from build123d import *

# Parameters (mm, degrees)
F0_W        = 88.9
F0_H        = 165.1
F1_DEPTH    = 6.35
F2_DEPTH    = 25.4
F3_DEPTH    = 50.8
F4_R        = 6.34999
F5_SIZE2    = 12.7
F5_SIZE     = 12.7
F6_C1_SIZE2 = 12.7
F6_C1_SIZE  = 7.3323484187
F6_C2_SIZE2 = 7.3323484187
F6_C2_SIZE  = 12.7
F6_C3_SIZE2 = 7.3323484187
F6_C3_SIZE  = 12.7
F6_C4_SIZE2 = 7.3323484187
F6_C4_SIZE  = 12.7


# Not quite as in the source:
# - a fillet or chamfer is up to 0.001 mm smaller than in the source, because OpenCascade refuses the exact size


with BuildPart() as f1:
    # F0 (on Top) → F1 (new body)
    with BuildSketch(Plane.XY):
        with Locations((59.7539862376, 23.8323401288)):
            Rectangle(F0_W, F0_H)
        Polygon((21.6539862376, 61.9323401288), (21.6539862376, 100.0323401288), (59.7539862376, 100.0323401288), (97.8539862376, 100.0323401288), (97.8539862376, -14.2676598712), (97.8539862376, -52.3676598712), (59.7539862376, -52.3676598712), (21.6539862376, -52.3676598712), align=None, mode=Mode.SUBTRACT)
    extrude(amount=F1_DEPTH)

    # F0 (on Top) → F2 (join)
    with BuildSketch(Plane.XY):
        with BuildLine():
            Line((97.8539862376, 100.0323401288), (59.7539862376, 100.0323401288))
            Line((59.7539862376, 100.0323401288), (59.7539862376, 74.6323401288))
            ThreePointArc((59.7539862376, 74.6323401288), (56.0342423587, 65.6520840077), (47.0539862376, 61.9323401288))
            Line((47.0539862376, 61.9323401288), (21.6539862376, 61.9323401288))
            Line((21.6539862376, 61.9323401288), (21.6539862376, -52.3676598712))
            Line((21.6539862376, -52.3676598712), (59.7539862376, -52.3676598712))
            Line((59.7539862376, -52.3676598712), (59.7539862376, -26.9676598712))
            ThreePointArc((59.7539862376, -26.9676598712), (63.4737301166, -17.9874037501), (72.4539862376, -14.2676598712))
            Line((72.4539862376, -14.2676598712), (97.8539862376, -14.2676598712))
            Line((97.8539862376, -14.2676598712), (97.8539862376, 100.0323401288))
        make_face()
    extrude(amount=F2_DEPTH)

    # F0 (on Top) → F3 (join)
    with BuildSketch(Plane.XY):
        with BuildLine():
            Line((59.7539862376, 100.0323401288), (21.6539862376, 100.0323401288))
            Line((21.6539862376, 100.0323401288), (21.6539862376, 61.9323401288))
            Line((21.6539862376, 61.9323401288), (47.0539862376, 61.9323401288))
            ThreePointArc((47.0539862376, 61.9323401288), (56.0342423587, 65.6520840077), (59.7539862376, 74.6323401288))
            Line((59.7539862376, 74.6323401288), (59.7539862376, 100.0323401288))
        make_face()
        with BuildLine():
            Line((97.8539862376, -52.3676598712), (97.8539862376, -14.2676598712))
            Line((97.8539862376, -14.2676598712), (72.4539862376, -14.2676598712))
            ThreePointArc((72.4539862376, -14.2676598712), (63.4737301166, -17.9874037501), (59.7539862376, -26.9676598712))
            Line((59.7539862376, -26.9676598712), (59.7539862376, -52.3676598712))
            Line((59.7539862376, -52.3676598712), (97.8539862376, -52.3676598712))
        make_face()
    extrude(amount=F3_DEPTH)

    # F4 (radius 6.35 in the source; OpenCascade refuses exactly that, so slightly less here)
    f4_edges = [f1.edges().sort_by_distance(p)[0] for p in [
        (15.303986, 23.83234, 6.35),
        (59.753986, 106.38234, 6.35),
        (59.753986, -58.71766, 6.35),
        (104.203986, 23.83234, 6.35),
    ]]
    fillet(f4_edges, radius=F4_R)

    # F5
    f5_edges = [f1.edges().sort_by_distance(p)[0] for p in [
        (21.653986, 4.78234, 25.4),
        (40.703986, -52.36766, 25.4),
        (97.853986, 42.88234, 25.4),
        (78.803986, 100.03234, 25.4),
    ]]
    chamfer(f5_edges, length=F5_SIZE, length2=F5_SIZE2)

    # F6: chamfer of 12.7 x 7.3323484187 on 4 edges, made by hand

    # F6_c1
    f6_c1_edges = [f1.edges().sort_by_distance(p)[0] for p in [
        (21.6539862376, 80.9823401288, 50.8),
    ]]
    f6_c1_side = f1.faces().sort_by_distance((21.6539862376, 80.9823401288, 50.6533530316))[0]
    chamfer(f6_c1_edges, length=F6_C1_SIZE, length2=F6_C1_SIZE2, reference=f6_c1_side)

    # F6_c2
    f6_c2_edges = [f1.edges().sort_by_distance(p)[0] for p in [
        (78.8039862376, -52.3676598712, 50.8),
    ]]
    f6_c2_side = f1.faces().sort_by_distance((78.8039862376, -52.3676598712, 50.6533530316))[0]
    chamfer(f6_c2_edges, length=F6_C2_SIZE, length2=F6_C2_SIZE2, reference=f6_c2_side)

    # F6_c3
    f6_c3_edges = [f1.edges().sort_by_distance(p)[0] for p in [
        (47.0539862376, 100.0323401288, 50.8),
    ]]
    f6_c3_side = f1.faces().sort_by_distance((47.0539862376, 100.0323401288, 50.6533530316))[0]
    chamfer(f6_c3_edges, length=F6_C3_SIZE, length2=F6_C3_SIZE2, reference=f6_c3_side)

    # F6_c4
    f6_c4_edges = [f1.edges().sort_by_distance(p)[0] for p in [
        (97.8539862376, -29.6514856618, 50.8),
    ]]
    f6_c4_side = f1.faces().sort_by_distance((97.8539862376, -29.6514856618, 50.6533530316))[0]
    chamfer(f6_c4_edges, length=F6_C4_SIZE, length2=F6_C4_SIZE2, reference=f6_c4_side)


solid = f1.part
Geometry: final body of the model. Coordinates: model frame, mm. A direction names the side the tool comes from. Round coordinates to 2 decimals unless told otherwise and drop trailing zeros. Order: outer loops, then holes, each group sorted by start corner. A loop starts at its lowest first (then second) coordinate and runs counter-clockwise, first axis right, second up. Notation, with made-up numbers: (-32, 47.25) -> (-18, 47.25) arc R6 ccw to (-18, 54.25) -> close; hole circle Ø10 at (45, 38). An arc over 180 degrees is marked (long way). Put each result on its own line as item: value. Start each with the question number.
Q1. Section D-D on z = 17.5. Return the cut outline in (x, y).
Q2. Line query: probe 1 along X at (y, z) = (-49.5, 35.5); probe 2 along X at (y, z) = (82.5, 26); probe 3 along Z at (x, y) = (98, 58.5). Output: solid intervals per line, ascending.
Q3. Section A-A on z = 36.5. Return the cut outline in (x, y).
Q4. Reachability of faces 1 (the flat face through (43, 100.032, 18)), 2 (the flat face through (76, -52.368, 18)), 3 (the flat face through (85, -14.268, 36)), 4 (the flat face through (21.654, 59, 12)), 5 (the flat face through (28.093, 5.582, 19.139)) from +Z, -Z, +X, -X, +Y, -Y: full face, straight path, thin tool, end or side. Return the list, or none.
Q5. First-contact query: pin 1 (3 mm diameter, centred on x = 26, y = -13, fed in from +Z); pin 2 (1 mm diameter, centred on y = -3.5, z = 9, fed in from -X); pin 3 (4 mm diameter, centred on x = 37, y = 22, fed in from -Z); pin 4 (12.5 mm diameter, centred on x = 81, z = 31, fed in from +Y). Flat tips, straight axial feed; report the tip coordinate or a pass-through.
Ans:
1. outline: (21.65, 61.93) -> (26.45, 61.93) -> (26.45, -47.57) -> (59.75, -47.57) -> (59.75, -52.37) -> (97.85, -52.37) -> (97.85, -14.27) -> (93.05, -14.27) -> (93.05, 95.23) -> (59.75, 95.23) -> (59.75, 100.03) -> (21.65, 100.03) -> close
2. probe 1: x = 59.75 to 97.85
2. probe 2: x = 21.65 to 59.75
2. probe 3: z = 0 to 6.35
3. outline: (21.65, 61.93) -> (47.05, 61.93) arc R12.7 ccw to (59.75, 74.63) -> (59.75, 100.03) -> (21.65, 100.03) -> close; (59.75, -52.37) -> (97.85, -52.37) -> (97.85, -14.27) -> (72.45, -14.27) arc R12.7 ccw to (59.75, -26.97) -> close
4. face 1: +Z, +X, -X, +Y
4. face 2: +Z, +X, -X, -Y
4. face 3: +Z, +X, +Y
4. face 4: +Z, -X, +Y, -Y
4. face 5: +Z, -X, -Y
5. pin 1: stops at z = 18.55
5. pin 2: stops at x = 21.65
5. pin 3: stops at z = 0
5. pin 4: stops at y = 87.98
